Part model, mm, in its own coordinate system. Round coordinates to 2 decimals unless told otherwise and drop trailing zeros. Loops run counter-clockwise (first coordinate to the right, second up) from the corner with the lowest first, then second, coordinate; pieces in that order, holes last. Notation, with made-up numbers: (73, -16.5) - (78, -16.5) arc R24 ccw to (78, 22.5) - close; hole circle Ø7 at (5.25, -35). An arc over 180 degrees is marked (long way). Put each result on its own line as item: value.
from build123d import *

# Parameters (mm, degrees)
SKETCH_1_R          = 60
SKETCH_1_R_2        = 25
EXTRUDE_1_DEPTH     = 5
SKETCH_2_R          = 1.8
CUT_EXTRUDE_1_DEPTH = 5
SKETCH_4_W          = 210
SKETCH_4_H          = 125
SKETCH_4_R          = 60
EXTRUDE_2_DEPTH     = 5
SKETCH_5_R          = 2.2
CUT_EXTRUDE_2_DEPTH = 5
FILLET_1_R          = 15


with BuildPart() as part:
    # 草图1 → 凸台-拉伸1 (new body)
    with BuildSketch(Plane(origin=(0, 0, 0), x_dir=(1, 0, 0), z_dir=(0, 1, 0))):
        with Locations(Location((0, 0, 0), (0, 0, 270))):
            Circle(SKETCH_1_R)
        with Locations(Location((0, 0, 0), (0, 0, 270))):
            Circle(SKETCH_1_R_2, mode=Mode.SUBTRACT)
    extrude(amount=EXTRUDE_1_DEPTH)

    # 草图2 → 切除-拉伸1 (cut)
    with BuildSketch(Plane(origin=(0, 5, 0), x_dir=(1, 0, 0), z_dir=(0, 1, 0))):
        with Locations(Location((0, 40, 0), (0, 0, 270))):
            Circle(SKETCH_2_R)
        with Locations(Location((40, 0, 0), (0, 0, 270))):
            Circle(SKETCH_2_R)
        with Locations(Location((0, -40, 0), (0, 0, 270))):
            Circle(SKETCH_2_R)
        with Locations(Location((-40, 0, 0), (0, 0, 270))):
            Circle(SKETCH_2_R)
    extrude(amount=-CUT_EXTRUDE_1_DEPTH, mode=Mode.SUBTRACT)

    # 草图4 → 凸台-拉伸2 (add)
    with BuildSketch(Plane(origin=(0, 0, 0), x_dir=(1, 0, 0), z_dir=(0, 1, 0))):
        Rectangle(SKETCH_4_W, SKETCH_4_H)
        Circle(SKETCH_4_R, mode=Mode.SUBTRACT)
    extrude(amount=EXTRUDE_2_DEPTH)

    # 草图5 → 切除-拉伸2 (cut)
    with BuildSketch(Plane(origin=(0, 5, 0), x_dir=(1, 0, 0), z_dir=(0, 1, 0))):
        with Locations(Location((-90, 47.5, 0), (0, 0, 270))):
            Circle(SKETCH_5_R)
        with Locations(Location((90, 47.5, 0), (0, 0, 90))):
            Circle(SKETCH_5_R)
        with Locations(Location((90, -47.5, 0), (0, 0, 270))):
            Circle(SKETCH_5_R)
        with Locations(Location((-90, -47.5, 0), (0, 0, 90))):
            Circle(SKETCH_5_R)
    extrude(amount=-CUT_EXTRUDE_2_DEPTH, mode=Mode.SUBTRACT)

    # 圆角1
    fillet_1_edges = [part.edges().sort_by_distance(p)[0] for p in [
        (-105, 2.5, -62.5),
        (-105, 2.5, 62.5),
        (105, 2.5, 62.5),
        (105, 2.5, -62.5),
    ]]
    fillet(fillet_1_edges, radius=FILLET_1_R)


solid = part.part
1. Band-saw the part on C-C (z = 6). List the corners of the cut face in (x, y), plus the area to 3 significant figures.
A:
outline: (-105, 0) - (-24.27, 0) - (-24.27, 5) - (-105, 5) - close; (24.27, 0) - (105, 0) - (105, 5) - (24.27, 5) - close
area: 807 mm²
2. Two-plate mould, pull along Z, no slides. Class faces 1 (the cylindrical face through (100.49, 2.54, 58.22)), 2 (the cylindrical face through (90.097, 2.535, 45.302)), 3 (the flat face through (-25, 0, -15)): pulls with the +Z half, pulls with the -Z half, needs draft (parallel to the pull), parting line crosses it, or undercut.
A:
face 1: pulls with the +Z half
face 2: undercut
face 3: needs draft
3. Band-saw the part on B-B (y = 1.3). Give the number of separate pieces and of enclosed holes in the cut face, plus the area to 3 significant figures.
A:
separate pieces: 1
enclosed holes: 9
area: 24,000 mm²
4. Probe line 1 along X through (y, z) = (1.7, 0); line 2 along X through (y, z) = (3.15, 40); line 3 along X through (y, z) = (1.85, 41). List the from-to ranges inside material, lowest first. Write a range as [from, to].
A:
line 1: x = [-105, -41.8], [-38.2, -25], [25, 38.2], [41.8, 105]
line 2: x = [-105, -1.8], [1.8, 105]
line 3: x = [-105, -1.5], [1.5, 105]
5. Band-saw the part on A-A (x = -10). List the corners of the cut face in (y, z), plus the area to 3 significant figures.
A:
outline: (0, -62.5) - (5, -62.5) - (5, -22.91) - (0, -22.91) - close; (0, 22.91) - (5, 22.91) - (5, 62.5) - (0, 62.5) - close
area: 396 mm²
